Autodesk Inventor part; units mm, degrees
ref_plane "YZ Plane" through (0, 0, 0) normal (1, 0, 0) x (0, 1, 0)
ref_plane "XZ Plane" through (0, 0, 0) normal (0, 1, 0) x (-1, 0, 0)
ref_plane "XY Plane" through (0, 0, 0) normal (0, 0, 1) x (1, 0, 0)
sketch "Sketch1" plane through (0, 0, 0) normal (0, 1, 0) x (-1, 0, 0)
  line L0 (0, 0) -> (152.4, 0)
  line L1 (152.4, 0) -> (152.4, 6.35)
  line L2 (34.925, 9.525) -> (3.175, 9.525)
  line L3 (0, 6.35) -> (0, 0)
  circle A0 centre (6.35, 4.7625) radius 2.5797
  circle A1 centre (31.75, 4.7625) radius 2.5797
  circle A2 centre (120.65, 4.7625) radius 2.5797
  circle A3 centre (146.05, 4.7625) radius 2.5797
  line L4 (38.1, 9.525) -> (114.3, 9.525)
  line L5 (114.3, 6.35) -> (114.3, 4.7625)
  line L6 (38.1, 4.7625) -> (38.1, 6.35)
  arc A4 (38.1, 6.35) -> (34.925, 9.525) centre (34.925, 6.35) ccw
  arc A5 (3.175, 9.525) -> (0, 6.35) centre (3.175, 6.35) ccw
  line L7 (117.475, 9.525) -> (149.225, 9.525)
  arc A6 (117.475, 9.525) -> (114.3, 6.35) centre (117.475, 6.35) ccw
  arc A7 (152.4, 6.35) -> (149.225, 9.525) centre (149.225, 6.35) ccw
  line L8 (114.3, 6.35) -> (114.3, 0)
  line L9 (38.1, 6.35) -> (38.1, 0)
  line L10 (114.3, 4.7625) -> (114.3, 9.525)
  line L11 (117.475, 9.525) -> (114.3, 9.525)
  line L12 (38.1, 6.35) -> (38.1, 9.525)
  line L13 (38.1, 9.525) -> (34.925, 9.525)
  line L14 (38.1, 3.175) -> (114.3, 3.175)
  point P0 (152.4, 9.525)
  point P1 (0, 9.525)
  dimension "d0" = 152.4
  dimension "d1" = 9.525
  dimension "d2" = 4.7625
  dimension "d3" = 4.7625
  dimension "d4" = 4.7625
  dimension "d5" = 4.7625
  dimension "d6" = 25.4
  dimension "d7" = 25.4
  dimension "d8" = 5.1594
  dimension "d9" = 6.35
  dimension "d10" = 6.35
  dimension "d11" = 4.7625
  dimension "d12" = 6.35
  dimension "d13" = 6.35
  dimension "d14" = 3.175
  dimension "d15" = 3.175
  dimension "d37" = 3.175
extrude "Extrusion1" add sketch "Sketch1" along normal mid plane 9.525 contours L3 A5 L2 A4 L6 L9 L0 | L9 L14 L8 L0 | L8 L5 A6 L7 A7 L1 L0
extrude "Extrusion2" add sketch "Sketch1" along normal mid plane 50.8 contours L9 L14 L8 L0
sketch "Sketch3" plane through (-152.4, -4.7625, 0) normal (0, 0, -1) x (-1, 0, 0)
  line L0 (-38.1, -20.6375) -> (-38.1, 0)
  line L1 (-114.3, 30.1625) -> (-38.1, 30.1625)
  line L2 (-38.1, 30.1625) -> (-38.1, -20.6375)
  line L3 (-38.1, -20.6375) -> (-114.3, -20.6375)
  line L4 (-114.3, -20.6375) -> (-114.3, 30.1625)
  circle A0 centre (-76.2, 4.7625) radius 9.525
  line L5 (-101.6, -20.6375) -> (-101.6, 30.1625)
  line L6 (-101.6, 30.1625) -> (-50.8, 30.1625)
  line L7 (-50.8, 30.1625) -> (-50.8, -20.6375)
  line L8 (-50.8, -20.6375) -> (-101.6, -20.6375)
  line L9 (-101.6, 17.4625) -> (-50.8, 17.4625)
  line L10 (-50.8, 17.4625) -> (-50.8, -7.9375)
  line L11 (-50.8, -7.9375) -> (-101.6, -7.9375)
  line L12 (-101.6, -7.9375) -> (-101.6, 17.4625)
  circle A1 centre (-101.6, 17.4625) radius 2.5797
  circle A2 centre (-101.6, -7.9375) radius 2.5797
  circle A3 centre (-50.8, -7.9375) radius 2.5797
  circle A4 centre (-50.8, 17.4625) radius 2.5797
  circle A5 centre (-101.6, 17.4625) radius 6.35
  circle A6 centre (-101.6, -7.9375) radius 6.35
  circle A7 centre (-50.8, -7.9375) radius 6.35
  circle A8 centre (-50.8, 17.4625) radius 6.35
  line L13 (-107.95, 23.8125) -> (-44.45, 23.8125)
  line L14 (-44.45, 23.8125) -> (-44.45, -14.2875)
  line L15 (-44.45, -14.2875) -> (-107.95, -14.2875)
  line L16 (-107.95, -14.2875) -> (-107.95, 23.8125)
  line L17 (-114.3, 9.525) -> (-117.475, 9.525)
  line L18 (-114.3, 0) -> (-114.3, 9.525)
  line L19 (-38.1, 0) -> (-38.1, 9.525)
  line L20 (-114.3, 9.525) -> (-107.95, 9.525)
  line L21 (-111.125, 9.525) -> (-101.3931, 37.1795)
  line L22 (-114.3, 0) -> (-114.3, 9.525)
  line L23 (-114.3, 0) -> (-107.95, 0)
  line L24 (-111.125, 0) -> (-100.7566, -29.4634)
  line L25 (-38.1, 0) -> (-44.45, 0)
  line L26 (-38.1, 9.525) -> (-38.1, 30.1625)
  line L27 (-38.1, 9.525) -> (-44.45, 9.525)
  line L28 (-41.275, 9.525) -> (-52.247, 40.7036)
  line L29 (-41.275, 0) -> (-51.6214, -29.4007)
  line L30 (0, 0) -> (-38.1, 0)
  line L31 (-114.3, 9.525) -> (-114.3, 30.1625)
  point P0 (-152.4, 4.7625)
  point P1 (-41.275, 0)
  point P2 (-107.5899, 19.5704)
  point P3 (-101.6, 23.8125)
  point P4 (-50.8, 23.8125)
  point P5 (-44.8101, 19.5704)
  point P6 (-38.1, 0)
  point P7 (-44.8101, -10.0454)
  point P8 (-50.8, -14.2875)
  point P9 (-101.6, -14.2875)
  point P10 (-107.5899, -10.0454)
  dimension "d38" = 25.4
  dimension "d39" = 38.1
  dimension "d40" = 50.8
  dimension "d41" = 25.4
  dimension "d42" = 12.7
  dimension "d43" = 19.05
  dimension "d44" = 5.1594
  dimension "d45" = 12.7
  dimension "d46" = 12.7
  dimension "d47" = 12.7
  dimension "d48" = 12.7
  dimension "d49" = 160.613
  dimension "d50" = 160.613
  dimension "d51" = 6.35
  dimension "d52" = 76.2
  dimension "d53" = 30.1625
  dimension "d54" = 13.5214
  dimension "d55" = 14.147
  dimension "d56" = 62.6566
  dimension "d57" = 63.2931
  dimension "d58" = 79.375
extrude "Extrusion4" cut sketch "Sketch3" against normal blind 50.8 contours L3 L29 L15 L14 L25 L0 | L3 L7 L15 L29 | L27 L28 L14 L13 L1 L2 | L3 L5 L15 L7 | L29 L14 L15 | L15 A7 L29 | L3 L24 L15 L5 | L28 L13 L7 L1 | L28 L13 L14 | L3 L4 L23 L24 L16 L15 | L15 L24 A6 | A3 L11 L7 | L7 A3 | L7 L13 L5 L1 | L28 A8 L13 | L15 L16 L24 | A2 L5 | L5 L11 A2 | L11 A3 L7 | L5 L13 L21 L1 | L5 A2 L11 | L21 L13 L16 L20 L4 L1 | A5 L21 L13 | A4 L7 | L7 L9 A4 | A4 L9 L7 | L21 L16 L13 | A1 L9 L5 | L5 A1 | L5 L9 A1 | A0
equation "\"d2\" = 0.5 * d1"
equation "\"d3\" = d2"
equation "\"d4\" = d2"
equation "\"d5\" = d2"
equation "\"d10\" = d9"
equation "\"d11\" = 0.5 * d1"
equation "\"d37\" = 0.333333 * d1"
properties part number "Face Plate"
Here's how the part is built. I have some questions about the finished solid (model axes, mm). A direction names the side the tool comes from. Give positions to 0.01 mm unless a question says otherwise; leave off trailing zeros. Loops run counter-clockwise (first coordinate to the right, second up) from the corner with the lowest first, then second, coordinate; pieces in that order, holes last. Notation, with made-up numbers: M 72.5,25.5 L 98.5,25.5 A25 cw 98.5,39.5 Z; hole C -25,16.5 d7. An arc over 180 degrees is marked long. Use one line per item in the form item = value. Start each with the question number.
Q1. If we section it at C-C (y = -8): Write out the boundary of the cut face in (x, z) (3 decimals), then the cut area to 3 significant figures.
Q2. I need wall thicknesses on line 1 along Y through (x, z) = (-51, 0.75); line 2 along X through (y, z) = (15, 0.75); line 3 along X through (y, z) = (3.5, 2.75). Which ranges of each line are inside material? Lowest first, please.
Q3. If we section it at D-D (x = -128): Write out the boundary of the cut face in (y, z) (1 decimal), then the cut area to 3 significant figures.
Q4. Which directions (+Z, -Z, +X, -X, +Y, -Y) give clear straight access to the entire face, cutting with the end or side of a thin tool? Please do faces 1 (the cylindrical face through (-37.145, -0.067, 8.62)), 2 (the flat face through (-132, -4.762, 5)), 3 (the flat face through (-131, 4.762, 5)), 4 (the cylindrical face through (-99.023, -12.587, 1.565)).
Q5. Thinking about a two-plate mould opening in X: for faces 5 (the flat face through (-114.3, 0, 5)), 6 (the flat face through (-20, 4.762, 5)), 7 (the cylindrical face through (-151.445, -0.067, 8.62)), 8 (the cylindrical face through (-148.433, -0.067, 5.751)), which applies, +X half, -X half, draft (parallel to the pull), parting line (faces both ways), or undercut?
Q6. Will these pins go through, and if not, where does the flat tip stop? pin 1 Ø3 at (x, z) = (-31.75, 4.76) entering from -Y; pin 2 Ø6.5 at (x, y) = (-101.6, 12.7) entering from +Z (3 decimals).
Q7. If we section it at A-A (y = 0): State how many separate pieces and enclosed holes the cut face has, then the cut area to 3 significant figures.
Q8. If we section it at B-B (x = -76.2): Write out the boundary of the cut face in (y, z) (3 decimals).
Taken from the geometry:
q1.outline = M -109.986,0 L -81.37,0 L -81.37,3.175 L -109.986,3.175 Z; M -71.03,0 L -42.414,0 L -42.414,3.175 L -71.03,3.175 Z
q1.area = 182 mm^2
q2.line_1 = -19.05 to -15.27, -10.13 to 10.13, 15.27 to 19.05
q2.line_2 = -107.52 to -102.77, -100.43 to -51.97, -49.63 to -44.88
q2.line_3 = -152.4 to -147.66, -144.44 to -122.26, -119.04 to -85.06, -67.34 to -33.36, -30.14 to -7.96, -4.74 to 0
q3.outline = M -4.8,0 L 4.8,0 L 4.8,9.5 L -4.8,9.5 Z
q3.area = 90.7 mm^2
q4.face_1 = +Z, +Y, -Y
q4.face_2 = +Z, -Z, -X, -Y
q4.face_3 = +Z, -Z, -X, +Y
q4.face_4 = +Z, -Z
q5.face_5 = undercut
q5.face_6 = draft
q5.face_7 = -X half
q5.face_8 = undercut
q6.pin_1 = through
q6.pin_2 = 3.175
q7.separate_pieces = 2
q7.enclosed_holes = 4
q7.area = 815 mm^2
q8.outline = M -19.05,0 L -9.525,0 L -9.525,3.175 L -19.05,3.175 Z; M 9.525,0 L 19.05,0 L 19.05,3.175 L 9.525,3.175 Z
